Input: part model. Units: mm. Frame: model coordinates. Face numbers are marked on the shaded views. A direction names the side the tool comes from. Coordinates: 2 decimals unless noted, no trailing zeros. Order: outer loops, then holes, each group sorted by start corner. A loop starts at its lowest first (then second) coordinate and runs counter-clockwise, first axis right, second up. Notation, with made-up numbers: (19, -6.75) - (41, -6.75) arc R19 ccw to (41, 26.25) - close; hole circle Ø10 at (32.5, 9). An arc over 180 degrees is marked (long way). Use a Markdown table: item, result. Add a question column.
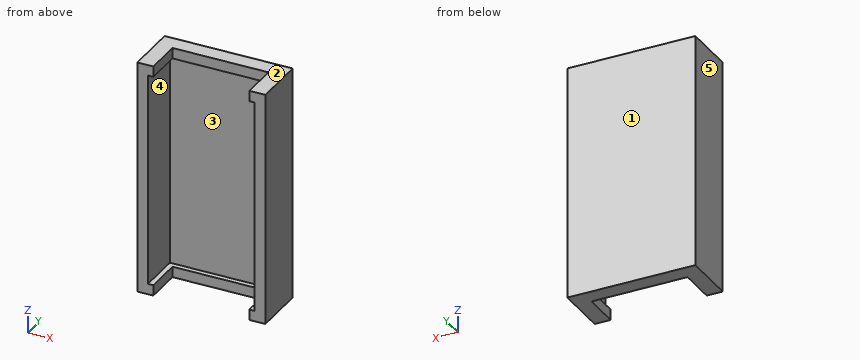
from build123d import *

# Parameters (mm, degrees)
F0_W     = 19.05
F0_H     = 34.925
F1_DEPTH = 7.9375
F2_W     = 15.875
F2_H     = 31.75
F3_DEPTH = 6.35
F4_W     = 14.2875
F4_H     = 5.55625
F5_DEPTH = 34.926


with BuildPart() as f1:
    # F0 (on Front) → F1 (new body)
    with BuildSketch(Plane.XZ):
        with Locations((-35.038067, 28.636673)):
            Rectangle(F0_W, F0_H)
    extrude(amount=F1_DEPTH)

    # F2 (on face) → F3 (cut)
    with BuildSketch(Plane.XZ.offset(7.9375)):
        with Locations((-35.038067, 28.636673)):
            Rectangle(F2_W, F2_H)
    extrude(amount=-F3_DEPTH, mode=Mode.SUBTRACT)

    # F4 (on face) → F5 (cut, through all)
    with BuildSketch(Plane.XY.offset(46.099173)):
        with Locations((-35.038067, -5.159375)):
            Rectangle(F4_W, F4_H)
    extrude(amount=-F5_DEPTH, mode=Mode.SUBTRACT)


solid = f1.part
1) Contact query for flat-ended pins moving along their axis: P1, Ø1, axis at x = -41.5, z = 25, coming from the -Y side; P2, Ø1.3, axis at x = -38.5, z = 12.5, coming from the -Y side; P3, Ø1.9, axis at x = -33.5, y = -3.5, coming from the +Z side. Output: stop coordinate, or through.
2) Cut plane C-C (z = 39). Return the cut outline in (x, y), and give its area (3 significant figures).
3) Cut plane B-B (x = -30). Return the cut outline in (y, z).
4) Pull-direction query (Z, two-part tool) for the marked faces 1, 2 and 3; classes: pulls with the +Z half, pulls with the -Z half, needs draft (parallel to the pull), parting line crosses it, or undercut.
5) Material intervals for L1, parallel to X at y = -6.75, z = 33.5; L2, parallel to Z at x = -33.25, y = -2; L3, parallel to Y at x = -31.25, z = 25, sorted ascending.
6) Reachability of the marked faces 4 and 5 from +Z, -Z, +X, -X, +Y, -Y: full face, straight path, thin tool, end or side. Return the list, or none.
7) Cut plane A-A (y = -4.25). Return the cut outline in (x, z), and give its area (3 significant figures).
Computed:
| question | item | result |
|---|---|---|
| 1 | P1 | stops at y = -1.59 |
| 1 | P2 | stops at y = -2.38 |
| 1 | P3 | passes through |
| 2 | outline | (-44.56, -7.94) - (-42.98, -7.94) - (-42.98, -1.59) - (-27.1, -1.59) - (-27.1, -7.94) - (-25.51, -7.94) - (-25.51, 0) - (-44.56, 0) - close |
| 2 | area | 50.4 mm2 |
| 3 | outline | (-2.38, 11.17) - (0, 11.17) - (0, 46.1) - (-2.38, 46.1) - (-2.38, 44.51) - (-1.59, 44.51) - (-1.59, 12.76) - (-2.38, 12.76) - close |
| 4 | face 1 | needs draft |
| 4 | face 2 | pulls with the +Z half |
| 4 | face 3 | undercut |
| 5 | L1 | x = -44.56 to -42.98, -27.1 to -25.51 |
| 5 | L2 | z = 11.17 to 12.76, 44.51 to 46.1 |
| 5 | L3 | y = -1.59 to 0 |
| 6 | face 4 | -Y |
| 6 | face 5 | +Z, -Z, -X, +Y, -Y |
| 7 | outline | (-44.56, 11.17) - (-42.18, 11.17) - (-42.18, 12.76) - (-42.98, 12.76) - (-42.98, 44.51) - (-42.18, 44.51) - (-42.18, 46.1) - (-44.56, 46.1) - close; (-27.89, 11.17) - (-25.51, 11.17) - (-25.51, 46.1) - (-27.89, 46.1) - (-27.89, 44.51) - (-27.1, 44.51) - (-27.1, 12.76) - (-27.89, 12.76) - close |
| 7 | area | 116 mm2 |
